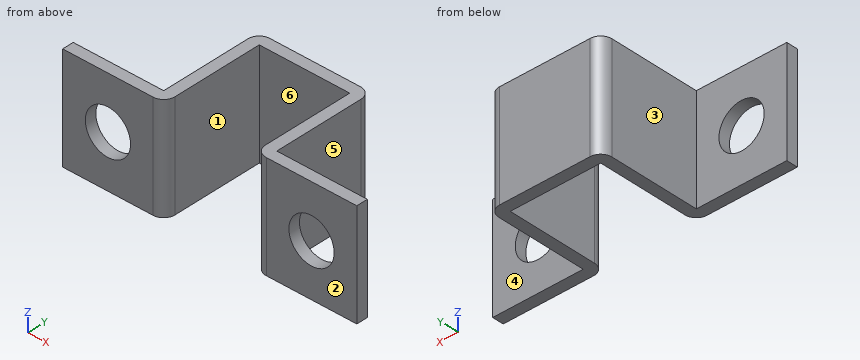
```python
from build123d import *

# Parameters (mm, degrees)
SM_START               = -7
SM_BASE_FLANGE_1_DEPTH = 14
SKETCH_6_R             = 3
CUT_EXTRUDE_1_DEPTH    = 10


# Read off the part's stored shape, not the designer's step: 基体-法兰1
with BuildPart() as part:
    # 基体-法兰1 outline → 基体-法兰1 (new body)
    with BuildSketch(Plane.XY.offset(SM_START)):
        with BuildLine():
            Line((7.5, -1.5), (19.5, -1.5))
            Line((19.5, -1.5), (19.5, 0))
            Line((19.5, 0), (7.5, 0))
            Line((7.5, 0), (7.5, 12))
            ThreePointArc((7.5, 12), (7.060660172, 13.060660172), (6, 13.5))
            Line((6, 13.5), (-6, 13.5))
            ThreePointArc((-6, 13.5), (-7.060660172, 13.060660172), (-7.5, 12))
            Line((-7.5, 12), (-7.5, 0))
            Line((-7.5, 0), (-19.5, 0))
            Line((-19.5, 0), (-19.5, -1.5))
            Line((-19.5, -1.5), (-7.5, -1.5))
            ThreePointArc((-7.5, -1.5), (-6.439339828, -1.060660172), (-6, 0))
            Line((-6, 0), (-6, 12))
            Line((-6, 12), (6, 12))
            Line((6, 12), (6, 0))
            ThreePointArc((6, 0), (6.439339828, -1.060660172), (7.5, -1.5))
        make_face()
    extrude(amount=SM_BASE_FLANGE_1_DEPTH)

    # 草图6 → 切除-拉伸1 (cut)
    with BuildSketch(Plane(origin=(0, 0, 0), x_dir=(1, 0, 0), z_dir=(0, 1, 0))):
        with Locations(Location((-13.5, 0, 0), (0, 0, 270))):
            Circle(SKETCH_6_R)
        with Locations(Location((13.5, 0, 0), (0, 0, 270))):
            Circle(SKETCH_6_R)
    extrude(amount=-CUT_EXTRUDE_1_DEPTH, mode=Mode.SUBTRACT)


solid = part.part
```
Source: CAD feature listing. Evaluate the final solid. Frame: model axes, mm. Face numbers are marked on the shaded views. A direction names the side the tool comes from. Give positions to 0.01 mm unless a question says otherwise; leave off trailing zeros. Write each loop counter-clockwise with the first axis right and the second up, starting at its lowest first coordinate (ties: lowest second). Pieces come first, ordered by that corner, then holes.
1. Material intervals for line 1 along X through (y, z) = (9, 0); line 2 along X through (y, z) = (-1, 0); line 3 along X through (y, z) = (-0.45, 0), sorted ascending.
2. Pull-direction query (X, two-part tool) for the marked faces 4, 5 and 6; classes: +X half, -X half, draft (parallel to the pull), parting line (faces both ways), or undercut.
3. First-contact query: pin 1 (3.5 mm diameter, centred on x = -15, z = 1.5, fed in from +Y); pin 2 (5 mm diameter, centred on x = -13.5, z = 0, fed in from +Y); pin 3 (6 mm diameter, centred on x = -2, z = -1.5, fed in from -Y); pin 4 (5 mm diameter, centred on x = 8.5, y = 11, fed in from -Z). Flat tips, straight axial feed; report the tip coordinate or a pass-through.
4. Access query for the marked faces 1, 2 and 3. Directions: +Z, -Z, +X, -X, +Y, -Y. A direction counts if a zero-diameter tool reaches every point of the face in a straight line with its end or side. Return the directions, or none.
5. Section query A-A (z = 0). Return the cut outline in (x, y).
6. Section query D-D (z = 4). Return the cut outline in (x, y).
7. Section query B-B (y = 0.5). Return the cut outline in (x, z).
8. Section query C-C (x = 13.5). Return the cut outline in (y, z).
Output values:
1. line 1: x = -7.5 to -6, 6 to 7.5
1. line 2: x = -19.5 to -16.5, -10.5 to -6.38, 6.38 to 10.5, 16.5 to 19.5
1. line 3: x = -19.5 to -16.5, -10.5 to -6.07, 6.07 to 10.5, 16.5 to 19.5
2. face 4: draft
2. face 5: +X half
2. face 6: undercut
3. pin 1: stops at y = 0
3. pin 2: passes through
3. pin 3: stops at y = 12
3. pin 4: stops at z = -7
4. face 1: +Z, -Z, -Y
4. face 2: +Z, -Z, +X, -X, -Y
4. face 3: +Z, -Z, -X, +Y
5. outline: (-19.5, -1.5) - (-16.5, -1.5) - (-16.5, 0) - (-19.5, 0) - close; (-10.5, -1.5) - (-7.5, -1.5) arc R1.5 ccw to (-6, 0) - (-6, 12) - (6, 12) - (6, 0) arc R1.5 ccw to (7.5, -1.5) - (10.5, -1.5) - (10.5, 0) - (7.5, 0) - (7.5, 12) arc R1.5 ccw to (6, 13.5) - (-6, 13.5) arc R1.5 ccw to (-7.5, 12) - (-7.5, 0) - (-10.5, 0) - close; (16.5, -1.5) - (19.5, -1.5) - (19.5, 0) - (16.5, 0) - close
6. outline: (-19.5, -1.5) - (-7.5, -1.5) arc R1.5 ccw to (-6, 0) - (-6, 12) - (6, 12) - (6, 0) arc R1.5 ccw to (7.5, -1.5) - (19.5, -1.5) - (19.5, 0) - (7.5, 0) - (7.5, 12) arc R1.5 ccw to (6, 13.5) - (-6, 13.5) arc R1.5 ccw to (-7.5, 12) - (-7.5, 0) - (-19.5, 0) - close
7. outline: (-7.5, -7) - (-6, -7) - (-6, 7) - (-7.5, 7) - close; (6, -7) - (7.5, -7) - (7.5, 7) - (6, 7) - close
8. outline: (-1.5, -7) - (0, -7) - (0, -3) - (-1.5, -3) - close; (-1.5, 3) - (0, 3) - (0, 7) - (-1.5, 7) - close
